Verification items for the finished model (mm, model axes). Round coordinates to 2 decimals unless told otherwise and drop trailing zeros. Loops run counter-clockwise (first coordinate to the right, second up) from the corner with the lowest first, then second, coordinate; pieces in that order, holes last. Notation, with made-up numbers: M -22.75,24.25 L 13.25,24.25 A18 cw 13.25,36.25 Z; hole C -7,-36 d6. An arc over 180 degrees is marked long. One line per item, written item: value.
from build123d import *

# Parameters (mm, degrees)
F0_W     = 117.799587
F0_H     = 65.169983
F1_DEPTH = 25.4
F2_SIZE  = 5.08
F3_R     = 9.441262
F4_DEPTH = 25.401


with BuildPart() as f1:
    # F0 (on Front) → F1 (new body)
    with BuildSketch(Plane.XZ):
        with Locations((-7.626143, 32.584992)):
            Rectangle(F0_W, F0_H)
    extrude(amount=F1_DEPTH)

    # F2
    f2_edges = [f1.edges().sort_by_distance(p)[0] for p in [
        (-66.525936, -12.7, 65.169983),
        (-7.626142, -25.4, 65.169983),
        (-66.525936, -25.4, 32.584991),
        (-7.626142, -25.4, 0),
        (51.273651, -25.4, 32.584991),
        (51.273651, -12.7, 65.169983),
    ]]
    chamfer(f2_edges, length=F2_SIZE)

    # F3 (on face) → F4 (cut, through all)
    with BuildSketch(Plane(origin=(0, 0, 0), x_dir=(-1, 0, 0), z_dir=(0, 1, 0))):
        with Locations((15.784286, 35.560001)):
            Circle(F3_R)
    extrude(amount=-F4_DEPTH, mode=Mode.SUBTRACT)


solid = f1.part
(1) Depth check by flat-ended pin: pin 1 Ø15 at (x, z) = (-15.78, 35.56) entering from -Y. Enter the tip coordinate at first touch or a pass-through.
Completed:
pin 1: passes through
(2) Thickness scan on L1, parallel to X at y = -18, z = 34.5; L2, parallel to Z at x = -24, y = -21.75; L3, parallel to Z at x = -21, y = -17.25. Record the ranges inside material, lowest first. Write a range as from..to.
Completed:
L1: x = -66.53..-25.17, -6.4..51.27
L2: z = 1.43..30.91, 40.21..63.74
L3: z = 0..27.69, 43.43..65.17
(3) Sectioned sample at B-B on y = -12.5. Enter the section's corners in (x, z).
Completed:
outline: M -66.53,0 L 51.27,0 L 51.27,60.09 L 46.19,65.17 L -61.45,65.17 L -66.53,60.09 Z; hole C -15.78,35.56 d18.88
(4) Mould release check, pull along X, two halves, no side actions. Record for faces 1 (the face through (-8.826, -12.522, 41.941)), 2 (the face through (48.134, -21.926, 61.624)), 3 (the face through (-8.38, -22.9, 62.59)), 4 (the face through (-63.95, -10.018, 62.666)): +X half, -X half, draft (parallel to the pull), parting line (faces both ways), or undercut.
Completed:
face 1: undercut
face 2: +X half
face 3: draft
face 4: -X half
(5) Sectioned sample at C-C on x = 20. Enter the section's corners in (y, z).
Completed:
outline: M -25.4,5.08 L -20.32,0 L 0,0 L 0,65.17 L -20.32,65.17 L -25.4,60.09 Z
(6) Sectioned sample at A-A on z = 35.56. Enter the section's corners in (x, y), and give its area (3 significant figures).
Completed:
outline: M -66.53,-20.32 L -61.45,-25.4 L -25.23,-25.4 L -25.23,0 L -66.53,0 Z; M -6.34,-25.4 L 46.19,-25.4 L 51.27,-20.32 L 51.27,0 L -6.34,0 Z
area: 2,490 mm^2
